Input: part model. Units: mm. Frame: model coordinates. A direction names the side the tool comes from. Round coordinates to 2 decimals unless told otherwise and drop trailing zeros. Loops run counter-clockwise (first coordinate to the right, second up) from the corner with the lowest first, then second, coordinate; pieces in that order, holes last.
(1) Line query: line 1 (Y direction, x = 0, z = 7.5); line 2 (Y direction, x = 0, z = -0.1). Output: solid intervals per line, ascending.
(2) Access query for faces 3 (the face through (-0.534, 4.065, 8.557)), 4 (the face through (3.233, -1.341, -0.007)). Directions: +Z, -Z, +X, -X, +Y, -Y. A direction counts if a zero-diameter tool reaches every point of the face in a straight line with its end or side. Return the directions, or none.
(3) Cut plane A-A, the plane z = 5. Output: boundary loops of the cut face in (x, y), and give its area (3 significant figures).
(4) Draft query along X for faces 1 (the face through (-0.534, 4.065, -8.76)), 2 (the face through (7.39, -3.06, 0.14)). Return one class per face: released by +X, released by -X, zero draft, split by the parting line, or undercut.
(5) First-contact query: pin 1 Ø5 at (x, y) = (6, -1) entering from -Z; pin 2 Ø3 at (x, z) = (-4.5, 12) entering from -Y; pin 3 Ø4 at (x, y) = (5.5, 6.5) entering from +Z; pin 4 Ø1 at (x, z) = (6, 5.5) entering from -Y. Flat tips, straight axial feed; report the tip coordinate or a pass-through.
from build123d import *

# Parameters (mm, degrees)
F0_R     = 4.1
F0_R_2   = 3.5
F1_DEPTH = 0.5
F0_R_3   = 8
F2_DEPTH = 16
F5_R     = 5


# Not quite as in the source:
# - a fillet or chamfer that OpenCascade refuses, or shapes differently, is made with other operations: its cross-section is extruded or revolved along the edge and cut away or added


with BuildPart() as f1:
    # F0 (on Top) → F1 (new body, symmetric)
    with BuildSketch(Plane.XY):
        Circle(F0_R)
        Circle(F0_R_2, mode=Mode.SUBTRACT)
    extrude(amount=F1_DEPTH, both=True)

    # F0 (on Top) → F2 (join, symmetric)
    with BuildSketch(Plane.XY):
        Circle(F0_R_3)
        Circle(F0_R, mode=Mode.SUBTRACT)
    extrude(amount=F2_DEPTH, both=True)

    # F3: fillet of radius 1 on 2 edges, made by hand

    # F3_s1 → F3_t2 (revolve)
    with BuildSketch(Plane.XZ):
        with BuildLine():
            ThreePointArc((4.1, 1.416515139), (3.9366600265, 0.8687925815), (3.5, 0.5))
            Line((3.5, 0.5), (4.1, 0.5))
            Line((4.1, 0.5), (4.1, 1.416515139))
        make_face()
    revolve(axis=Axis((0, 0, 0.5), (0, 0, 1)))

    # F3_s3 → F3_t4 (revolve)
    with BuildSketch(Plane.XZ):
        with BuildLine():
            ThreePointArc((4.1, -1.416515139), (3.9366600265, -0.8687925815), (3.5, -0.5))
            Line((3.5, -0.5), (4.1, -0.5))
            Line((4.1, -0.5), (4.1, -1.416515139))
        make_face()
    revolve(axis=Axis((0, 0, -0.5), (0, 0, 1)))

    # F4: chamfer of 4 on 2 edges, made by hand

    # F4_s1 → F4_t2 (revolve, cut)
    with BuildSketch(Plane.XZ):
        Polygon((8, -12), (4, -16), (8, -16), align=None)
    revolve(axis=Axis((0, 0, -16), (0, 0, 1)), mode=Mode.SUBTRACT)

    # F4_s3 → F4_t4 (revolve, cut)
    with BuildSketch(Plane.XZ):
        Polygon((8, 12), (4, 16), (8, 16), align=None)
    revolve(axis=Axis((0, 0, 16), (0, 0, 1)), mode=Mode.SUBTRACT)

    # F5
    f5_edges = [f1.edges().sort_by_distance(p)[0] for p in [
        (-8, 0, -12),
        (-8, 0, 12),
    ]]
    fillet(f5_edges, radius=F5_R)


solid = f1.part
Reported:
1. line 1: y = -8 to -4.1, 4.1 to 8
1. line 2: y = -8 to -3.5, 3.5 to 8
2. face 3: +Z
2. face 4: +Z, -Z
3. outline: circle Ø16 at (0, 0); hole circle Ø8.2 at (0, 0)
3. area: 148 mm2
4. face 1: undercut
4. face 2: split by the parting line
5. pin 1: stops at z = -15.9
5. pin 2: stops at y = -7.14
5. pin 3: stops at z = 13.49
5. pin 4: stops at y = -5.81
